from build123d import *

# Parameters (mm, degrees)
F1_DEPTH      = 19.05
F3_DEPTH      = 228.6
F5_DEPTH      = 203.2
F5_DEPTH_BACK = 1676.4
F6_W          = 38.1
F6_H          = 9.525
F7_DEPTH      = 203.2
F8_W          = 1219.2
F8_H          = 914.4
F9_DEPTH      = 25.4
F10_W         = 600.075
F10_H         = 901.7
F11_DEPTH     = 19.05


with BuildPart() as f1:
    # F0 (on Top) → F1 (new body)
    with BuildSketch(Plane.XY):
        Polygon((0, 228.6), (0, 0), (95.25, 0), (298.45, 171.45), (298.45, 228.6), align=None)
    extrude(amount=F1_DEPTH)

    # F2 (on face) → F3 (join)
    with BuildSketch(Plane.XZ):
        Polygon((38.1, 0), (0, 0), (0, -38.1), (38.1, -38.1), (76.2, -38.1), (76.2, -19.05), (38.1, -19.05), align=None)
    extrude(amount=-F3_DEPTH)

    # F4 (on face) → F5 (join, two sides)
    with BuildSketch(Plane.YZ.offset(298.45)) as f5_sk:
        Polygon((190.5, 0), (171.45, 0), (171.45, -38.1), (190.5, -38.1), (190.5, -28.575), (228.6, -28.575), (228.6, -9.525), (190.5, -9.525), align=None)
    extrude(amount=-F5_DEPTH)
    extrude(f5_sk.sketch, amount=F5_DEPTH_BACK)

    # F6 (on face) → F7 (join)
    with BuildSketch(Plane.YZ.offset(298.45)):
        with Locations((209.55, -4.7625)):
            Rectangle(F6_W, F6_H)
    extrude(amount=-F7_DEPTH)

    # F8 (on face) → F9 (join)
    with BuildSketch(Plane.XZ.offset(-171.45)):
        with Locations((1289.05, -19.05)):
            Rectangle(F8_W, F8_H)
    extrude(amount=F9_DEPTH)

    # F10 (on face) → F11 (cut)
    with BuildSketch(Plane(origin=(0, 171.45, 0), x_dir=(-1, 0, 0), z_dir=(0, 1, 0))):
        with Locations((-1592.2625, -19.05)):
            Rectangle(F10_W, F10_H)
        with Locations((-985.8375, -19.05)):
            Rectangle(F10_W, F10_H)
    extrude(amount=-F11_DEPTH, mode=Mode.SUBTRACT)


solid = f1.part
Geometry: final body of the model. Coordinates: model frame, mm. A direction names the side the tool comes from. Give positions to 0.01 mm unless a question says otherwise; leave off trailing zeros. Write each loop counter-clockwise with the first axis right and the second up, starting at its lowest first coordinate (ties: lowest second). Pieces come first, ordered by that corner, then holes.
(1) Cut plane C-C, the plane y = 23. Return loops of the section in (x, z).
(2) Mould query, pull axis Y, two halves, no side actions, for faces 1 (the flat face through (383, 171.45, -19)), 2 (the flat face through (38, 113, -38.1)), 3 (the flat face through (1286.2, 171.45, 220.1)), 4 (the flat face through (990, 171.45, -19)). Classes: released by +Y, released by -Y, zero draft, split by the parting line, or undercut.
(3) Cut plane D-D, the plane x = 331.5. Return loops of the section in (y, z) (3 decimals).
(4) Cut plane B-B, the plane z = 339. Return loops of the section in (x, y) (3 decimals), then the cut area to 3 significant figures.
(5) Ray query, line 1 (X direction, y = 218, z = -23); line 2 (Y direction, x = 743, z = -101); line 3 (Z direction, x = 1673, y = 171.5). Return the intervals inside material, ascending.
(6) First-contact query: P1, Ø3, axis at y = 149.5, z = 95, coming from the +X side; P2, Ø5.5, axis at x = 935.5, y = 177, coming from the +Z side; P3, Ø15, axis at x = 1218, y = 183, coming from the -Z side. Flat tips, straight axial feed; report the tip coordinate or a pass-through.
(7) Cut plane A-A, the plane x = 1255. Return loops of the section in (y, z) (3 decimals).
(8) Access query for faces 5 (the flat face through (138, 116, 0)), 6 (the flat face through (95.25, 200, -15)), 7 (the flat face through (1022, 209, -28.575)), 8 (the flat face through (114, 141, 19.05)), 9 (the flat face through (1125, 210, -9.525)). Directions: +Z, -Z, +X, -X, +Y, -Y. A direction counts if a zero-diameter tool reaches every point of the face in a straight line with its end or side. Return the directions, or none.
Values follow:
1. outline: (0, -38.1) - (76.2, -38.1) - (76.2, -19.05) - (38.1, -19.05) - (38.1, 0) - (122.51, 0) - (122.51, 19.05) - (0, 19.05) - close
2. face 1: released by -Y
2. face 2: zero draft
2. face 3: released by +Y
2. face 4: undercut
3. outline: (171.45, -38.1) - (190.5, -38.1) - (190.5, -28.575) - (228.6, -28.575) - (228.6, -9.525) - (190.5, -9.525) - (190.5, 0) - (171.45, 0) - close
4. outline: (679.45, 146.05) - (1898.65, 146.05) - (1898.65, 171.45) - (1892.3, 171.45) - (1892.3, 152.4) - (1292.225, 152.4) - (1292.225, 171.45) - (1285.875, 171.45) - (1285.875, 152.4) - (685.8, 152.4) - (685.8, 171.45) - (679.45, 171.45) - close
4. area: 8,100 mm2
5. line 1: x = 0 to 76.2, 95.25 to 1974.85
5. line 2: y = 146.05 to 152.4
5. line 3: z = -38.1 to 0
6. P1: stops at x = 1898.65
6. P2: stops at z = 0
6. P3: stops at z = -38.1
7. outline: (146.05, -476.25) - (171.45, -476.25) - (171.45, -469.9) - (152.4, -469.9) - (152.4, 431.8) - (171.45, 431.8) - (171.45, 438.15) - (146.05, 438.15) - close; (171.45, -38.1) - (190.5, -38.1) - (190.5, -28.575) - (228.6, -28.575) - (228.6, -9.525) - (190.5, -9.525) - (190.5, 0) - (171.45, 0) - close
8. face 5: -Y
8. face 6: -Z, +Y, -Y
8. face 7: -Z, +X, +Y
8. face 8: +Z, -X, +Y, -Y
8. face 9: +Z, +X, +Y
